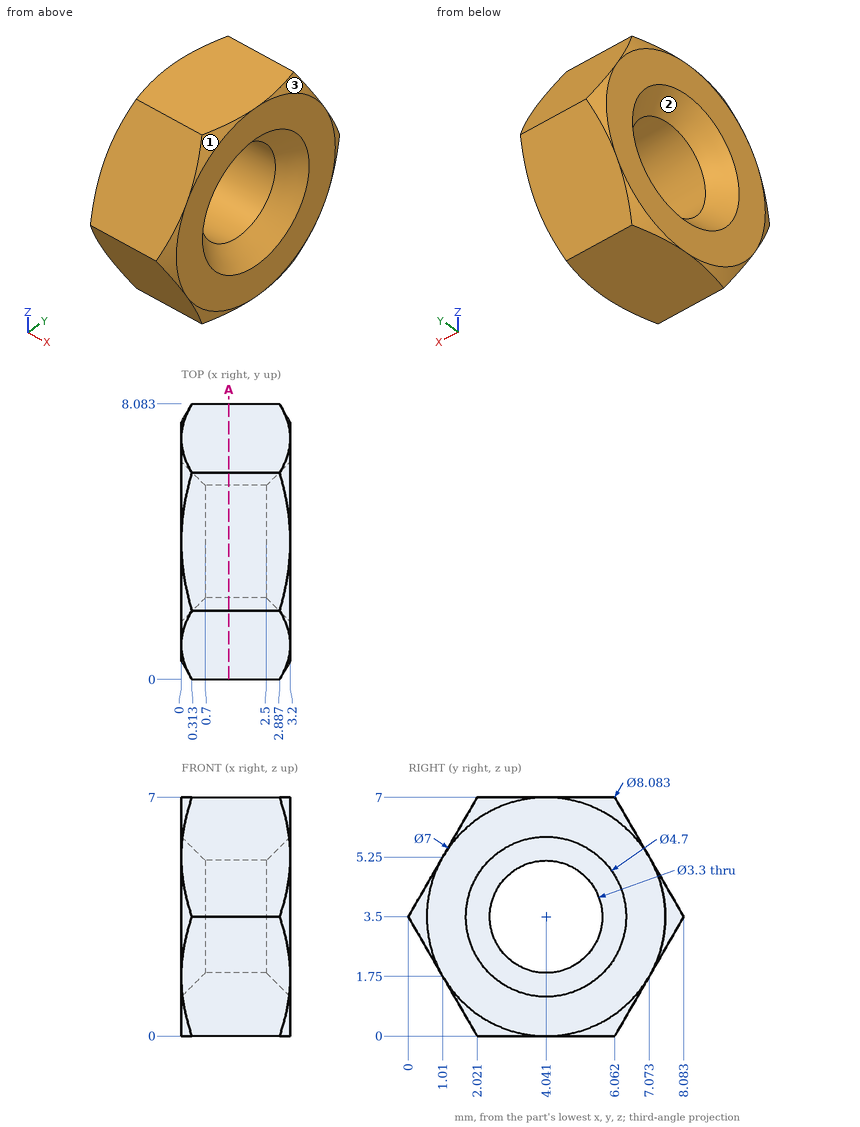
Verification items for this drawing (mm, ordinates from the low corner). Give positions to 0.01 mm unless a question says otherwise; leave off trailing zeros. Loops run counter-clockwise (first coordinate to the right, second up) from the corner with the lowest first, then second, coordinate; pieces in that order, holes last. Notation, with made-up numbers: M -8.5,15 L 4.5,15 A12 ccw 4.5,19 Z; hole C 34.5,-24 d3. An arc over 180 degrees is marked long. Write item = value, one per line.
(1) Release check for a two-part mould opening along Y. For the marked faces 1, 2 and 3 record: released by +Y, released by -Y, zero draft, split by the parting line, or undercut.
Answer below:
face_1 = released by -Y
face_2 = undercut
face_3 = released by +Y
(2) Sectioned sample at A-A, the plane x = 1.4. Record the cut outline in (y, z).
Answer below:
outline = M 0,3.5 L 2.02,0 L 6.06,0 L 8.08,3.5 L 6.06,7 L 2.02,7 Z; hole C 4.04,3.5 d3.3
(3) Gauge pin test, flat end, axial feed: pin 1 Ø1 at (x, z) = (1, 1) entering from +Y. Record the tip position at first contact, or that the pin passes through.
Answer below:
pin_1 = 6.93
(4) Material ranges on line 1 (Z direction, x = 2.8, y = 4.5) (1 decimal); line 2 (Z direction, x = 1.35, y = 3); line 3 (Y direction, x = 0.2, z = 6.25) (1 decimal), recorded low to high. Write a range as [from, to].
Answer below:
line_1 = [0, 1.6], [5.4, 7]
line_2 = [0, 2.22], [4.78, 7]
line_3 = [1.6, 6.5]
